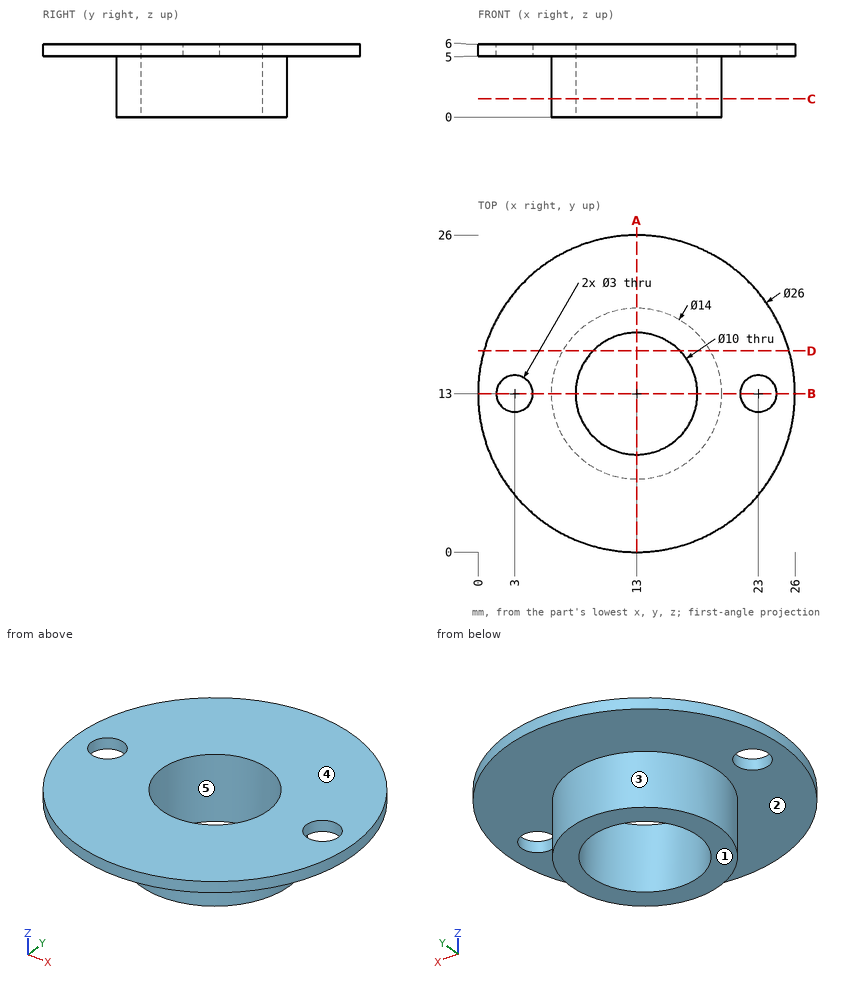
Job drawing, mm, ordinate dimensions from the low corner. One solid piece. A direction names the side the tool comes from. Coordinates: 2 decimals unless noted, no trailing zeros. Write each loop counter-clockwise with the first axis right and the second up, starting at its lowest first coordinate (ties: lowest second). Pieces come first, ordered by that corner, then holes.
Item 1: Probe line 1 (Z direction, x = 22.5, y = 7.25); line 2 (Y direction, x = 3, z = 5.6); line 3 (Y direction, x = 9.75, z = 4.8). List the from-to ranges inside material, lowest first.
Item 2: Slice it at A-A (x = 13). Write the cut outline in (y, z).
Item 3: Slice it at C-C (z = 1.5). Write the cut outline in (x, y).
Item 4: Slice it at D-D (y = 16.5). Write the cut outline in (x, z), and give its area (3 significant figures).
Item 5: Which spindle directions (+Z, -Z, +X, -X, +Y, -Y) get a long thin tool onto all of the face, cutting with end or side? Do the marked faces 1 and 2. Say none if no direction does.
Item 6: Slice it at B-B (y = 13). Write the cut outline in (x, z).
Item 7: Mould opens along X. For the marked faces 3, 4 and 5 say: released by +X, released by -X, zero draft, split by the parting line, or undercut.
Item 8: Pin check, flat tips, straight feed: pin 1 (1.5 mm diameter, centred on y = 17, z = 3, fed in from +X); pin 2 (3 mm diameter, centred on x = 7, z = 1.5, fed in from +Y). Stop position of each tip, or through.
Results found:
1. line 1: z = 5 to 6
1. line 2: y = 4.69 to 11.5, 14.5 to 21.31
1. line 3: y = 6.8 to 9.2, 16.8 to 19.2
2. outline: (0, 5) - (6, 5) - (6, 0) - (8, 0) - (8, 6) - (0, 6) - close; (18, 0) - (20, 0) - (20, 5) - (26, 5) - (26, 6) - (18, 6) - close
3. outline: circle Ø14 at (13, 13); hole circle Ø10 at (13, 13)
4. outline: (0.48, 5) - (6.94, 5) - (6.94, 0) - (9.43, 0) - (9.43, 6) - (0.48, 6) - close; (16.57, 0) - (19.06, 0) - (19.06, 5) - (25.52, 5) - (25.52, 6) - (16.57, 6) - close
4. area: 42.8 mm2
5. face 1: -Z, +X, -X, +Y, -Y
5. face 2: -Z
6. outline: (0, 5) - (1.5, 5) - (1.5, 6) - (0, 6) - close; (4.5, 5) - (6, 5) - (6, 0) - (8, 0) - (8, 6) - (4.5, 6) - close; (18, 0) - (20, 0) - (20, 5) - (21.5, 5) - (21.5, 6) - (18, 6) - close; (24.5, 5) - (26, 5) - (26, 6) - (24.5, 6) - close
7. face 3: split by the parting line
7. face 4: zero draft
7. face 5: undercut
8. pin 1: stops at x = 19.2
8. pin 2: stops at y = 18.36
